Check sheet for the modelled part. Datum: model origin and axes. Units: mm. Face numbers are marked on the shaded views. A direction names the side the tool comes from. Give positions to 0.01 mm unless a question says otherwise; leave off trailing zeros. Write each loop counter-clockwise with the first axis right and the second up, starting at its lowest first coordinate (ties: lowest second). Pieces come first, ordered by that corner, then holes. Notation, with made-up numbers: (81.25, 34) -> (85.25, 34) arc R25 ccw to (85.25, 59) -> close; hole circle Ø2 at (-35.5, 46.5). An arc over 180 degrees is marked (long way). Answer as a JSON object with one key per item and string values.
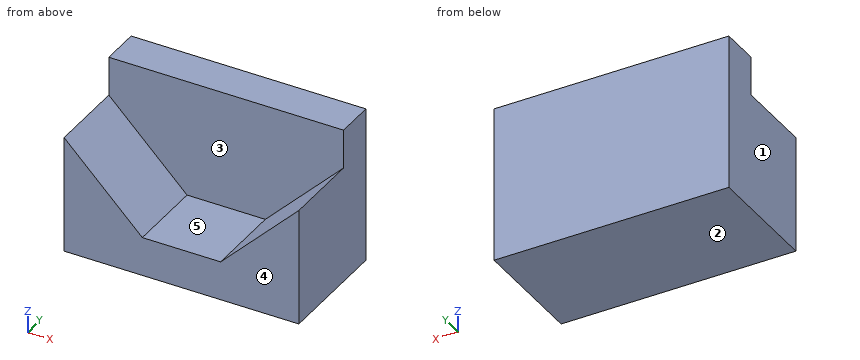
from build123d import *

# Parameters (mm, degrees)
F0_W     = 152.4
F0_H     = 76.2
F1_DEPTH = 101.6
F2_W     = 50.8
F2_H     = 25.4
F3_DEPTH = 152.4
F5_DEPTH = 50.8


with BuildPart() as f1:
    # F0 (on Top) → F1 (new body)
    with BuildSketch(Plane.XY):
        with Locations((1.659449, -35.339441)):
            Rectangle(F0_W, F0_H)
    extrude(amount=F1_DEPTH)

    # F2 (on face) → F3 (cut)
    with BuildSketch(Plane.YZ.offset(77.859449)):
        with Locations((-48.039441, 88.9)):
            Rectangle(F2_W, F2_H)
    extrude(amount=-F3_DEPTH, mode=Mode.SUBTRACT)

    # F4 (on face) → F5 (cut)
    with BuildSketch(Plane.XZ.offset(73.439441)):
        Polygon((77.859449, 76.2), (27.059449, 76.2), (27.059449, 41.245621), (27.059449, 25.4), align=None)
        Polygon((27.059449, 76.2), (-23.740551, 76.2), (-23.740551, 25.4), (27.059449, 25.4), (27.059449, 41.245621), align=None)
        Polygon((-23.740551, 76.2), (-74.540551, 76.2), (-23.740551, 25.4), align=None)
    extrude(amount=-F5_DEPTH, mode=Mode.SUBTRACT)


solid = f1.part
1. Access from +Z, -Z, +X, -X, +Y, -Y to the whole of each face (thin tool, end or side, straight path). Record for the marked faces 4 and 5.
Determined:
{"face 4": "+Z, -Z, +X, -X, -Y", "face 5": "+Z, -Y"}
2. Go/stop test with flat-tipped pins: P1, Ø6, axis at x = 30, y = -32, coming from the +Z side; P2, Ø6, axis at x = 29, z = 38, coming from the -Y side. Record where each tip stops, or that it passes through.
Determined:
{"P1": "z = 31.34", "P2": "y = -22.64"}
3. Mould release check, pull along X, two halves, no side actions. Record for the marked faces 1, 2 and 3: released by +X, released by -X, zero draft, split by the parting line, or undercut.
Determined:
{"face 1": "released by -X", "face 2": "zero draft", "face 3": "undercut"}
4. Sectioned sample at B-B, the plane z = 57. Enter the section's corners in (x, y), plus the area to 3 significant figures.
Determined:
{"outline": "(-74.54, -73.44) -> (-55.34, -73.44) -> (-55.34, -22.64) -> (58.66, -22.64) -> (58.66, -73.44) -> (77.86, -73.44) -> (77.86, 2.76) -> (-74.54, 2.76) -> close", "area": "5,820 mm^2"}
5. Sectioned sample at A-A, the plane x = 15. Enter the section's corners in (y, z).
Determined:
{"outline": "(-73.44, 0) -> (2.76, 0) -> (2.76, 101.6) -> (-22.64, 101.6) -> (-22.64, 25.4) -> (-73.44, 25.4) -> close"}
6. Scan lines: L1, parallel to Y at x = 24, z = 55; L2, parallel to Z at x = 17.5, y = -35; L3, parallel to X at y = -57.5, z = 30.5. Record each from-to range of solid material in increasing order. Write a range as [from, to].
Determined:
{"L1": "[-22.64, 2.76]", "L2": "[0, 25.4]", "L3": "[-74.54, -28.84], [32.16, 77.86]"}
7. Sectioned sample at C-C, the plane y = -37. Enter the section's corners in (x, z), plus the area to 3 significant figures.
Determined:
{"outline": "(-74.54, 0) -> (77.86, 0) -> (77.86, 76.2) -> (27.06, 25.4) -> (-23.74, 25.4) -> (-74.54, 76.2) -> close", "area": "6,450 mm^2"}
8. Sectioned sample at D-D, the plane z = 39. Enter the section's corners in (x, y), plus the area to 3 significant figures.
Determined:
{"outline": "(-74.54, -73.44) -> (-37.34, -73.44) -> (-37.34, -22.64) -> (40.66, -22.64) -> (40.66, -73.44) -> (77.86, -73.44) -> (77.86, 2.76) -> (-74.54, 2.76) -> close", "area": "7,650 mm^2"}
